from build123d import *

# Parameters (mm, degrees)
SKETCH2_W                = 400
SKETCH2_H                = 290
BASE_FLANGE1_DEPTH       = 3.175
CUT_EXTRUDE1_DEPTH       = 10
M6_CLEARANCE_HOLE1_D     = 6.6
M6_CLEARANCE_HOLE1_DEPTH = 18.75
M6_CLEARANCE_HOLE1_TIP   = 1.982840043


# Sheet-metal steps are written as plain solids
with BuildPart() as part:
    # Sketch2 (on Top Plane) → Base-Flange1 (new body)
    with BuildSketch(Plane(origin=(0, 0, 0), x_dir=(1, 0, 0), z_dir=(0, 1, 0))):
        Rectangle(SKETCH2_W, SKETCH2_H)
    extrude(amount=-BASE_FLANGE1_DEPTH)

    # Sketch10 → Cut-Extrude1 (cut)
    with BuildSketch(Plane(origin=(0, 0, 0), x_dir=(1, 0, 0), z_dir=(0, 1, 0))):
        Polygon((200, 68.8), (200, 145), (123.8, 145), align=None)
        Polygon((-200, 145), (-123.8, 145), (-200, 68.8), align=None)
    extrude(amount=-CUT_EXTRUDE1_DEPTH, mode=Mode.SUBTRACT)

    # M6 Clearance Hole1
    with Locations(Plane(origin=(0, 0, 0), x_dir=(1, 0, 0), z_dir=(0, 1, 0))):
        with Locations((-187.3, -132.3), (187.3, -132.3), (116.467651581, 132.3), (-116.467651581, 132.3)):
            Hole(M6_CLEARANCE_HOLE1_D / 2, depth=M6_CLEARANCE_HOLE1_DEPTH)
            with Locations((0, 0, -(M6_CLEARANCE_HOLE1_DEPTH + M6_CLEARANCE_HOLE1_TIP / 2))):  # 118° drill point
                Cone(0, M6_CLEARANCE_HOLE1_D / 2, M6_CLEARANCE_HOLE1_TIP, mode=Mode.SUBTRACT)


solid = part.part
Verification items for the finished model (mm, model axes). Round coordinates to 2 decimals unless told otherwise and drop trailing zeros. Write each loop counter-clockwise with the first axis right and the second up, starting at its lowest first coordinate (ties: lowest second). Pieces come first, ordered by that corner, then holes.
(1) Depth check by flat-ended pin: pin 1 Ø8.5 at (x, z) = (-187.3, 132.3) entering from -Y (3 decimals). Enter the tip coordinate at first touch or a pass-through.
Returned:
pin 1: stops at y = -3.175
(2) Section check B-B (x = 165). Enter the section's corners in (y, z) (3 decimals), plus the area to 3 significant figures.
Returned:
outline: (-3.175, -103.8) - (0, -103.8) - (0, 145) - (-3.175, 145) - close
area: 790 mm2
(3) Material ranges on line 1 (X direction, y = -2.4, z = 133); line 2 (X direction, y = -0.95, z = 132.3); line 3 (Z direction, x = 187.3, y = -2), recorded low to high.
Returned:
line 1: x = -200 to -190.52, -184.08 to 184.08, 190.52 to 200
line 2: x = -200 to -190.6, -184 to 184, 190.6 to 200
line 3: z = -81.5 to 129, 135.6 to 145
(4) Section check A-A (y = -2.3). Enter the section's corners in (x, z), plus the area to 3 significant figures.
Returned:
outline: (-200, -68.8) - (-123.8, -145) - (123.8, -145) - (200, -68.8) - (200, 145) - (-200, 145) - close; hole circle Ø6.6 at (-187.3, 132.3); hole circle Ø6.6 at (-116.47, -132.3); hole circle Ø6.6 at (116.47, -132.3); hole circle Ø6.6 at (187.3, 132.3)
area: 110,000 mm2
